Part print with two shaded views. Sizes in mm from the minimum x, y, z corner. A direction names the side the tool comes from. Give positions to 0.01 mm unless a question says otherwise; leave off trailing zeros. Loops run counter-clockwise (first coordinate to the right, second up) from the corner with the lowest first, then second, coordinate; pieces in that order, holes last. Notation, with made-up numbers: (17, 40) -> (52, 40) arc R9 cw to (52, 46) -> close; hole circle Ø2 at (66.5, 13.5). An arc over 180 degrees is marked (long way). One line per question, with ' | ' between items.
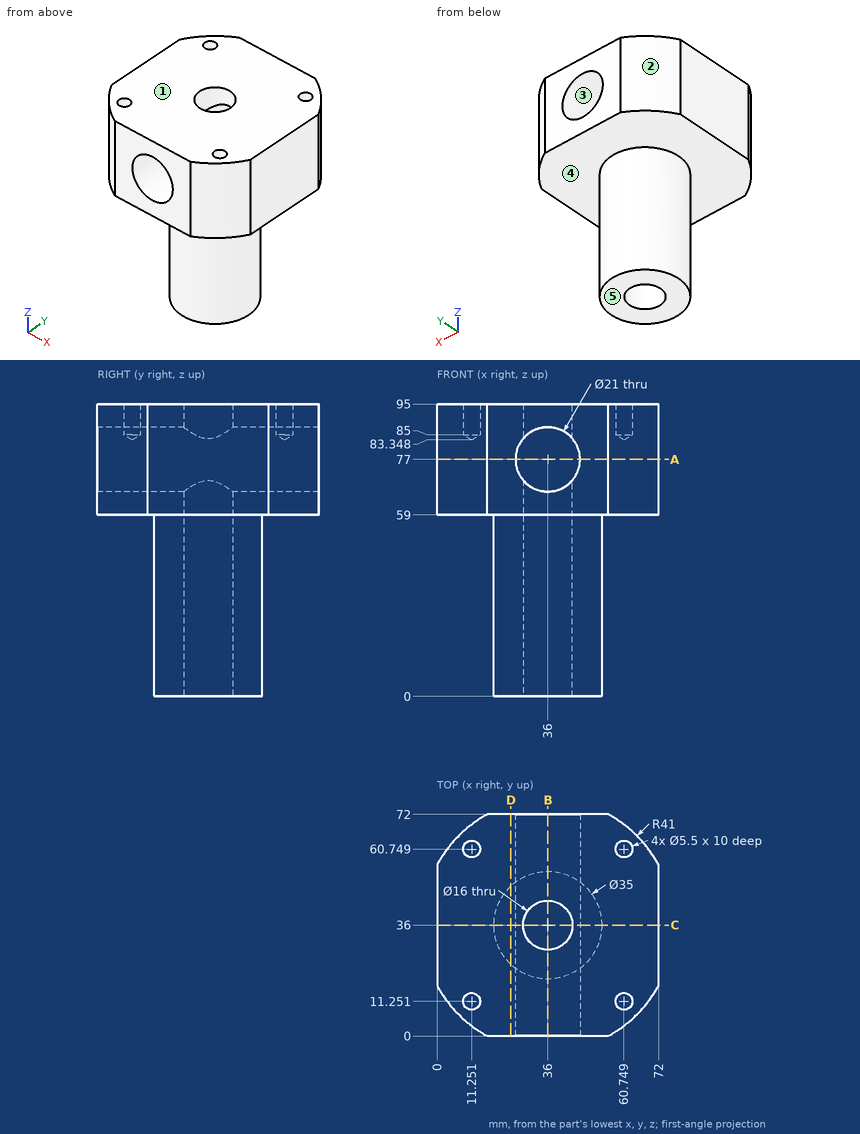
1) Drill centre lines: line 1 (Z direction, x = 21.5, y = 60); line 2 (Y direction, x = 29, z = 45.5) (1 decimal); line 3 (Z direction, x = 39, y = 64.5). Where is each one in solid material? Low to high.
Found:
line 1: 59 to 95 | line 2: 20 to 32.1, 39.9 to 52 | line 3: 59 to 66.94, 87.06 to 95
2) Saw through at D-D (x = 24). Give the cut face in (y, z).
Found:
outline: (0, 59) -> (23.26, 59) -> (23.26, 0) -> (48.74, 0) -> (48.74, 59) -> (72, 59) -> (72, 95) -> (0, 95) -> close
3) Tool access for the marked faces 4 and 5: list every direction of +Z, -Z, +X, -X, +Y, -Y with a clear straight run to the whole face (end or side of a thin tool).
Found:
face 4: -Z | face 5: -Z, +X, -X, +Y, -Y
4) Pin check, flat tips, straight feed: P1, Ø6, axis at y = 17.5, z = 43, coming from the -X side (1 decimal); P2, Ø4, axis at y = 53.5, z = 22.5, coming from the +X side (1 decimal); P3, Ø1.5, axis at y = 22, z = 43, coming from the -X side. Stop position of each tip, or through.
Found:
P1: x = 27.9 | P2: x = 44.1 | P3: x = 24.57
5) Saw through at C-C (y = 36). Give the cut face in (x, z).
Found:
outline: (0, 59) -> (18.5, 59) -> (18.5, 0) -> (28, 0) -> (28, 70.2) arc R10.5 cw to (28, 83.8) -> (28, 95) -> (0, 95) -> close; (44, 0) -> (53.5, 0) -> (53.5, 59) -> (72, 59) -> (72, 95) -> (44, 95) -> (44, 83.8) arc R10.5 cw to (44, 70.2) -> close
6) Pull direction X, two halves, no side cores. Call the marked faces 1, 2 and 3: pulls with the +X half, pulls with the -X half, needs draft (parallel to the pull), parting line crosses it, or undercut.
Found:
face 1: needs draft | face 2: pulls with the -X half | face 3: undercut
7) Saw through at A-A (z = 77). Give the cut face in (x, y).
Found:
outline: (0, 16.38) arc R41 ccw to (16.38, 0) -> (25.5, 0) -> (25.5, 72) -> (16.38, 72) arc R41 ccw to (0, 55.62) -> close; (46.5, 0) -> (55.62, 0) arc R41 ccw to (72, 16.38) -> (72, 55.62) arc R41 ccw to (55.62, 72) -> (46.5, 72) -> close
8) Saw through at B-B (x = 36). Give the cut face in (y, z), and give its area (3 significant figures).
Found:
outline: (0, 59) -> (18.5, 59) -> (18.5, 0) -> (28, 0) -> (28, 66.5) -> (0, 66.5) -> close; (0, 87.5) -> (28, 87.5) -> (28, 95) -> (0, 95) -> close; (44, 0) -> (53.5, 0) -> (53.5, 59) -> (72, 59) -> (72, 66.5) -> (44, 66.5) -> close; (44, 87.5) -> (72, 87.5) -> (72, 95) -> (44, 95) -> close | area: 1,960 mm2
